Check sheet for the modelled part. Datum: model origin and axes. Units: mm. A direction names the side the tool comes from. Give positions to 0.01 mm unless a question says otherwise; leave off trailing zeros. Write each loop counter-clockwise with the first axis right and the second up, starting at its lowest first coordinate (ties: lowest second). Pieces come first, ordered by that corner, then holes. Notation, with made-up numbers: (65.5, 86) -> (109.5, 86) arc R22 cw to (109.5, 116) -> close; hole circle Ø5 at (54, -28). An arc over 180 degrees is marked (long way). Answer as a JSON object with one key per item and string values.
from build123d import *

# Parameters (mm, degrees)
SM_BASE_FLANGE_1_DEPTH            = 2.91
CUT_EXTRUDE_START                 = -9.92
CUT_EXTRUDE_2_OUTLINE_W           = 5
CUT_EXTRUDE_2_OUTLINE_H           = 0.71
CUT_EXTRUDE_2_DEPTH               = 9.52
CUT_EXTRUDE_START_2               = -0.4
CUT_EXTRUDE_2_2_OUTLINE_W         = 0.9
CUT_EXTRUDE_2_2_OUTLINE_H         = 0.71
CUT_EXTRUDE_2_2_DEPTH             = 0.4
SM_EDGE_FLANGE_2_STRIP_W          = 1.8
SM_EDGE_FLANGE_2_STRIP_H          = 0.4
SM_EDGE_FLANGE_2_STRIP_CUT_DEPTH  = 0.63
SM_EDGE_FLANGE_2_RELIEF_W         = 1.98
SM_EDGE_FLANGE_2_RELIEF_H         = 0.8
SM_EDGE_FLANGE_2_RELIEF_CUT_DEPTH = 0.4
SM_EDGE_FLANGE_2_DEPTH            = 0.63
FILLET_3_R                        = 0.18
CUT_EXTRUDE_4_DEPTH               = 12.348755283
FILLET_4_R                        = 1
SKETCH_33_W                       = 2.00295296
SKETCH_33_H                       = 3.384867517
CUT_EXTRUDE_5_DEPTH               = 13.417670735


# Read off the part's stored shape, not the designer's step: 切除-拉伸2
# Sheet-metal steps are written as plain solids
with BuildPart() as part:
    # Sketch 1 → 基体-法兰1 (new body)
    with BuildSketch(Plane.XY):
        with BuildLine():
            Line((-3.4172, 3.19), (-2.64194931, 2.466293544))
            ThreePointArc((-2.64194931, 2.466293544), (-2.338641394, 1.90383514), (-2.437847629, 1.272556064))
            ThreePointArc((-2.437847629, 1.272556064), (-2.730725187, -0.325023008), (-2.071040526, -1.809223905))
            ThreePointArc((-2.071040526, -1.809223905), (-1.841158131, -2.283453933), (-1.884290869, -2.808696355))
            Line((-1.884290869, -2.808696355), (-2.689927651, -5.025447504))
            ThreePointArc((-2.689927651, -5.025447504), (-2.712424525, -5.109527023), (-2.72, -5.196233927))
            Line((-2.72, -5.196233927), (-2.72, -5.83))
            ThreePointArc((-2.72, -5.83), (-2.573553391, -6.183553391), (-2.22, -6.33))
            Line((-2.22, -6.33), (0, -6.33))
            Line((0, -6.33), (0, -6.73))
            Line((0, -6.73), (-2.22, -6.73))
            ThreePointArc((-2.22, -6.73), (-2.856396103, -6.466396103), (-3.12, -5.83))
            Line((-3.12, -5.83), (-3.12, -5.196233927))
            ThreePointArc((-3.12, -5.196233927), (-3.106364145, -5.0401615), (-3.065869772, -4.888818365))
            Line((-3.065869772, -4.888818365), (-2.26023299, -2.672067216))
            ThreePointArc((-2.26023299, -2.672067216), (-2.234353348, -2.356921763), (-2.372282784, -2.072383746))
            ThreePointArc((-2.372282784, -2.072383746), (-3.127921577, -0.372299082), (-2.792443648, 1.457655128))
            ThreePointArc((-2.792443648, 1.457655128), (-2.732919907, 1.836422573), (-2.914904656, 2.173897616))
            Line((-2.914904656, 2.173897616), (-3.690155347, 2.897604072))
            Line((-3.690155347, 2.897604072), (-3.4172, 3.19))
        make_face()
    extrude(amount=SM_BASE_FLANGE_1_DEPTH)

    # 切除-拉伸2 outline → 切除-拉伸2 (cut)
    with BuildSketch(Plane.XZ.offset(6.73).offset(CUT_EXTRUDE_START)):
        with Locations((-2.5, 2.555)):
            Rectangle(CUT_EXTRUDE_2_OUTLINE_W, CUT_EXTRUDE_2_OUTLINE_H)
    extrude(amount=CUT_EXTRUDE_2_DEPTH, mode=Mode.SUBTRACT)

    # Cut-Extrude 2 2 outline → Cut-Extrude 2 2 (cut)
    with BuildSketch(Plane.XZ.offset(6.73).offset(CUT_EXTRUDE_START_2)):
        with Locations((-2.67, 2.555)):
            Rectangle(CUT_EXTRUDE_2_2_OUTLINE_W, CUT_EXTRUDE_2_2_OUTLINE_H)
    extrude(amount=CUT_EXTRUDE_2_2_DEPTH, mode=Mode.SUBTRACT)

    # 边线-法兰2 strip (across the edge) → 边线-法兰2 strip cut (cut)
    with BuildSketch(Plane(origin=(0, -6.73, 2.91), x_dir=(0, 0, -1), z_dir=(-1, 0, 0))):
        with Locations((-0.4, -0.2)):
            Rectangle(SM_EDGE_FLANGE_2_STRIP_W, SM_EDGE_FLANGE_2_STRIP_H)
    extrude(amount=SM_EDGE_FLANGE_2_STRIP_CUT_DEPTH, mode=Mode.SUBTRACT)

    # 边线-法兰2 relief (on the sheet) → 边线-法兰2 relief cut (cut)
    with BuildSketch(Plane(origin=(0, -6.73, 2.41), x_dir=(0, 0, -1), z_dir=(0, -1, 0))):
        with Locations((-0.81, -1.03)):
            Rectangle(SM_EDGE_FLANGE_2_RELIEF_W, SM_EDGE_FLANGE_2_RELIEF_H)
    extrude(amount=-SM_EDGE_FLANGE_2_RELIEF_CUT_DEPTH, mode=Mode.SUBTRACT)

    # 边线-法兰2 section (across the edge) → 边线-法兰2 (add)
    with BuildSketch(Plane(origin=(0, -6.73, 2.91), x_dir=(0, 0, -1), z_dir=(-1, 0, 0))):
        with BuildLine():
            Line((0, 0.1), (0, 3.6))
            Line((0, 3.6), (0.4, 3.6))
            Line((0.4, 3.6), (0.4, 0.1))
            ThreePointArc((0.4, 0.1), (0.429289322, 0.029289322), (0.5, 0))
            Line((0.5, 0), (0.5, -0.4))
            ThreePointArc((0.5, -0.4), (0.146446609, -0.253553391), (0, 0.1))
        make_face()
    extrude(amount=SM_EDGE_FLANGE_2_DEPTH)

    # 圆角3
    fillet_3_edges = [part.edges().sort_by_distance(p)[0] for p in [
        (-1.43, -6.53, 2.23),
        (-0.63, -6.53, 2.23),
    ]]
    fillet(fillet_3_edges, radius=FILLET_3_R)

    # 草图29 → 切除-拉伸4 (cut, through all)
    with BuildSketch(Plane.XY.offset(2.91)):
        with BuildLine():
            Line((-0.63, -8.93), (-1.33273135, -8.93))
            Line((-1.33273135, -8.93), (-1.33273135, -10.562100009))
            Line((-1.33273135, -10.562100009), (0, -10.562100009))
            Line((0, -10.562100009), (0, -10.33))
            ThreePointArc((0, -10.33), (-0.465244282, -9.697609927), (-0.63, -8.93))
        make_face()
    extrude(amount=-CUT_EXTRUDE_4_DEPTH, mode=Mode.SUBTRACT)

    # 圆角4
    fillet_4_edges = [part.edges().sort_by_distance(p)[0] for p in [
        (-3.553677673, 3.043802036, 2.2),
    ]]
    fillet(fillet_4_edges, radius=FILLET_4_R)

    # 镜向8: part across plane


with BuildPart() as part_1:
    add(part.part)
    add(part.part.mirror(Plane(origin=(0, -6.33, 2.91), x_dir=(0, 0, 1), z_dir=(1, 0, 0))))

    # 镜向9: part across plane


with BuildPart() as part_2:
    add(part_1.part)
    add(part_1.part.mirror(Plane(origin=(-2.26023299, -2.672067216, 0), x_dir=(1, 0, 0), z_dir=(0, 0, -1))))

    # 草图33 → 切除-拉伸5 (cut, through all)
    with BuildSketch(Plane.XY.offset(2.91)):
        with Locations((0, -9.272433759)):
            Rectangle(SKETCH_33_W, SKETCH_33_H)
    extrude(amount=-CUT_EXTRUDE_5_DEPTH, mode=Mode.SUBTRACT)


solid = part_2.part
1. Sectioned sample at A-A, the plane y = 0. Enter the section's corners in (x, z), plus the area to 3 significant figures.
Determined:
{"outline": "(-3.15, -2.2) -> (-2.75, -2.2) -> (-2.75, 2.2) -> (-3.15, 2.2) -> close; (2.75, -2.2) -> (3.15, -2.2) -> (3.15, 2.2) -> (2.75, 2.2) -> close", "area": "3.52 mm^2"}
2. Scan lines: L1, parallel to Y at x = 1.5, z = -2.2; L2, parallel to X at y = -5.5, z = -0.35; L3, parallel to X at y = -3.5, z = 0.7. Record each from-to range of solid material in increasing order. Write a range as [from, to].
Determined:
{"L1": "[-6.73, -6.33]", "L2": "[-3.12, -2.72], [2.72, 3.12]", "L3": "[-2.56, -2.14], [2.14, 2.56]"}
3. Go/stop test with flat-tipped pins: P1, Ø1.5, axis at x = -0.5, y = 1.5, coming from the -Z side; P2, Ø2, axis at y = -6, z = -2, coming from the -X side; P3, Ø0.7, axis at y = -5.5, z = 0, coming from the +X side; P4, Ø1.5, axis at x = 2, z = 2, coming from the -Y side. Record where each tip stops, or that it passes through.
Determined:
{"P1": "through", "P2": "x = -3.12", "P3": "x = 3.12", "P4": "y = -6.73"}
4. Sectioned sample at B-B, the plane x = -0.5. Enter the section's corners in (y, z).
Determined:
{"outline": "(-7.58, -2.91) -> (-6.83, -2.91) arc R0.5 ccw to (-6.33, -2.41) -> (-6.33, 2.41) arc R0.5 ccw to (-6.83, 2.91) -> (-7.58, 2.91) -> (-7.58, 2.51) -> (-6.83, 2.51) arc R0.1 cw to (-6.73, 2.41) -> (-6.73, -2.41) arc R0.1 cw to (-6.83, -2.51) -> (-7.58, -2.51) -> close"}
5. Mould release check, pull along X, two halves, no side actions. Record for faces 1 (the face through (2.34, -1.75, -2.2)), 2 (the face through (-3.125, -0.399, 0.031)), 3 (the face through (2.85, -6.47, 0.03)), 4 (the face through (-2.733, -0.302, 0.031)): released by +X, released by -X, zero draft, split by the parting line, or undercut.
Determined:
{"face 1": "zero draft", "face 2": "released by -X", "face 3": "released by +X", "face 4": "undercut"}
6. Access from +Z, -Z, +X, -X, +Y, -Y to the whole of each face (thin tool, end or side, straight path). Record for faces 5 (the face through (-2.67, -3.8, 0.03)), 6 (the face through (-2.28, -3.9, 0.03)), 7 (the face through (3.332, 2.841, -1.915)).
Determined:
{"face 5": "+Z, -Z, -X", "face 6": "+Z, -Z", "face 7": "-Z, +X, +Y"}
7. Sectioned sample at C-C, the plane y = -3.5. Enter the section's corners in (x, z), plus the area to 3 significant figures.
Determined:
{"outline": "(-2.56, -2.2) -> (-2.14, -2.2) -> (-2.14, 2.2) -> (-2.56, 2.2) -> close; (2.14, -2.2) -> (2.56, -2.2) -> (2.56, 2.2) -> (2.14, 2.2) -> close", "area": "3.75 mm^2"}
